```python
from build123d import *

# Parameters (mm, degrees)
BOSS_EXTRU_1_DEPTH      = 4
ESQUISSE2_R             = 1
ESQUISSE2_W             = 29.690189182
ESQUISSE2_H             = 17.433113391
ENL_V_MAT_EXTRU_1_DEPTH = 4
ESQUISSE4_W             = 18
ESQUISSE4_H             = 24
ENL_V_MAT_EXTRU_2_DEPTH = 10


with BuildPart() as part:
    # Esquisse1 → Boss.-Extru.1 (new body)
    with BuildSketch(Plane(origin=(0, 0, 0), x_dir=(1, 0, 0), z_dir=(0, 1, 0))):
        with BuildLine():
            Line((-16.1, 0), (-16.1, -113.9))
            Line((-16.1, -113.9), (16.1, -113.9))
            Line((16.1, -113.9), (16.1, 0))
            ThreePointArc((16.1, 0), (0, 16.1), (-16.1, 0))
        make_face()
    extrude(amount=BOSS_EXTRU_1_DEPTH)

    # Esquisse2 → Enlèv. mat.-Extru.1 (cut)
    with BuildSketch(Plane(origin=(0, 4, 0), x_dir=(1, 0, 0), z_dir=(0, 1, 0))):
        with Locations(Location((-13.5, -92.9, 0), (0, 0, 270))):
            Circle(ESQUISSE2_R)
        with Locations(Location((-13.5, -100.9, 0), (0, 0, 270))):
            Circle(ESQUISSE2_R)
        with Locations(Location((13.5, -92.9, 0), (0, 0, 270))):
            Circle(ESQUISSE2_R)
        with Locations(Location((13.5, -100.9, 0), (0, 0, 270))):
            Circle(ESQUISSE2_R)
        with Locations(Location((13.5, -108.9, 0), (0, 0, 270))):
            Circle(ESQUISSE2_R)
        with Locations(Location((-13.5, -108.9, 0), (0, 0, 270))):
            Circle(ESQUISSE2_R)
        with Locations(Location((13.154905409, -4.448481213, 0), (0, 0, 270))):
            Circle(ESQUISSE2_R)
        with Locations(Location((-13.845094591, 3.551518787, 0), (0, 0, 270))):
            Circle(ESQUISSE2_R)
        with Locations(Location((-13.845094591, -4.448481213, 0), (0, 0, 270))):
            Circle(ESQUISSE2_R)
        with Locations(Location((13.154905409, 3.551518787, 0), (0, 0, 270))):
            Circle(ESQUISSE2_R)
        with Locations((0, 14.948183015)):
            Rectangle(ESQUISSE2_W, ESQUISSE2_H)
    extrude(amount=-ENL_V_MAT_EXTRU_1_DEPTH, mode=Mode.SUBTRACT)

    # Esquisse4 → Enlèv. mat.-Extru.2 (cut)
    with BuildSketch(Plane(origin=(0, 4, 0), x_dir=(1, 0, 0), z_dir=(0, 1, 0))):
        with Locations((0.316024011, -101.9)):
            Rectangle(ESQUISSE4_W, ESQUISSE4_H)
    extrude(amount=-ENL_V_MAT_EXTRU_2_DEPTH, mode=Mode.SUBTRACT)


solid = part.part
```
Can you work these out from the model? Positions are in its coordinate system, mm. A direction names the side the tool comes from. Give positions to 0.01 mm unless a question says otherwise; leave off trailing zeros. Loops run counter-clockwise (first coordinate to the right, second up) from the corner with the lowest first, then second, coordinate; pieces in that order, holes last. Notation, with made-up numbers: M 73.25,12.25 L 129.25,12.25 A17 cw 129.25,28.25 Z; hole C 1.25,-35.75 d5. An arc over 180 degrees is marked long. Answer in a Markdown table with one row per item.
1. If I drill on line 1 along X through (y, z) = (1.7, 108.9); line 2 along Z through (x, y) = (8.5, 0.4); line 3 along X through (y, z) = (1.1, 103.5), over which ranges is the centre line in solid material (lowest first)?
Taken from the geometry:
| item | result |
|---|---|
| line 1 | x = -16.1 to -14.5, -12.5 to -8.68, 9.32 to 12.5, 14.5 to 16.1 |
| line 2 | z = -6.23 to 89.9 |
| line 3 | x = -16.1 to -8.68, 9.32 to 16.1 |
2. Suppose I cut it at B-B on y = 1.1. Count the separate pieces of the cut face and the enclosed holes in it, plus the area to 3 significant figures.
Taken from the geometry:
| item | result |
|---|---|
| separate pieces | 1 |
| enclosed holes | 10 |
| area | 3,400 mm² |
3. Suppose I cut it at C-C on x = 4.5. Write out the boundary of the cut face in (y, z).
Taken from the geometry:
| item | result |
|---|---|
| outline | M 0,-6.23 L 4,-6.23 L 4,89.9 L 0,89.9 Z |
4. Suppose I cut it at A-A on z = 92.9. Write out the boundary of the cut face in (x, y), plus the area to 3 significant figures.
Taken from the geometry:
| item | result |
|---|---|
| outline | M -16.1,0 L -14.5,0 L -14.5,4 L -16.1,4 Z; M -12.5,0 L -8.68,0 L -8.68,4 L -12.5,4 Z; M 9.32,0 L 12.5,0 L 12.5,4 L 9.32,4 Z; M 14.5,0 L 16.1,0 L 16.1,4 L 14.5,4 Z |
| area | 40.8 mm² |
5. Which directions (+Z, -Z, +X, -X, +Y, -Y) give clear straight access to the entire face, cutting with the end or side of a thin tool? Please do faces 5 (the cylindrical face through (12.9, 2, 108.1)), 6 (the flat face through (9.316, 2, 102)).
Taken from the geometry:
| item | result |
|---|---|
| face 5 | +Y, -Y |
| face 6 | +Z, +Y, -Y |
6. Thinking about a two-plate mould opening in X: for faces 1 (the flat face through (-16.1, 2, 56)), 2 (the cylindrical face through (15.8, 2, -3.1)), 3 (the flat face through (0, 2, 89.9)), 4 (the flat face through (-12, 2, 113.9)), which applies, released by +X, released by -X, zero draft, split by the parting line, or undercut?
Taken from the geometry:
| item | result |
|---|---|
| face 1 | released by -X |
| face 2 | released by +X |
| face 3 | undercut |
| face 4 | zero draft |
